from build123d import *

# Parameters (mm, degrees)
MAKERBEAMFIX_DEPTH              = 15
SKETCH3_W                       = 30
SKETCH3_H                       = 12
SKETCH3_R                       = 3.25
SKETCH3_R_2                     = 4.5
DRILLKEYANDSMALLHEXDRIVER_DEPTH = 10
SKETCH4_R                       = 1.5
FIXINGHOLE_DEPTH                = 15
SKETCH5_R                       = 4.25
DRIVERHOLE_DEPTH                = 7


with BuildPart() as part:
    # Sketch1 → MakerBeamFix (new body, symmetric)
    with BuildSketch(Plane.XY):
        Polygon((-5, 0), (5, 0), (5, 1), (1.45, 1), (1.45, 2), (-1.45, 2), (-1.45, 1), (-5, 1), align=None)
    extrude(amount=MAKERBEAMFIX_DEPTH, both=True)

    # Sketch3 → DrillKeyAndSmallHexDriver (add)
    with BuildSketch(Plane.ZY.offset(5)):
        with Locations((0, -6)):
            Rectangle(SKETCH3_W, SKETCH3_H)
        with Locations((9, -6)):
            Circle(SKETCH3_R, mode=Mode.SUBTRACT)
        with Locations((-8, -6)):
            Circle(SKETCH3_R_2, mode=Mode.SUBTRACT)
    extrude(amount=-DRILLKEYANDSMALLHEXDRIVER_DEPTH)

    # Sketch4 → FixingHole (cut, through all)
    with BuildSketch(Plane.XZ.offset(12)):
        with Locations((0, 1)):
            Circle(SKETCH4_R)
    extrude(amount=-FIXINGHOLE_DEPTH, mode=Mode.SUBTRACT)

    # Sketch5 → DriverHole (cut, through all)
    with BuildSketch(Plane(origin=(0, -6, 0), x_dir=(1, 0, 0), z_dir=(0, 1, 0))):
        with Locations((0, -1)):
            Circle(SKETCH5_R)
    extrude(amount=-DRIVERHOLE_DEPTH, mode=Mode.SUBTRACT)


solid = part.part
Geometry: final body of the model. Coordinates: model frame, mm. A direction names the side the tool comes from. Round coordinates to 2 decimals unless told otherwise and drop trailing zeros. Loops run counter-clockwise (first coordinate to the right, second up) from the corner with the lowest first, then second, coordinate; pieces in that order, holes last. Notation, with made-up numbers: (83.25, 38.25) - (139.25, 38.25) arc R21 ccw to (139.25, 69.25) - close; hole circle Ø8 at (86.5, 50.25). An arc over 180 degrees is marked (long way). Write each question's results on one line, items separated by ' | '. Start each with the question number.
1) Cut plane C-C on y = -7.75. Return loops of the section in (x, z), then the cut area to 3 significant figures.
2) Cut plane B-B on z = 1. Return loops of the section in (x, y), then the cut area to 3 significant figures.
3) Cut plane D-D on z = -8. Return loops of the section in (x, y).
4) Line query: probe 1 along Z at (x, y) = (0.5, -7.25); probe 2 along Z at (x, y) = (-4, -4.5); probe 3 along Z at (x, y) = (0.5, -8.25). Output: solid intervals per line, ascending. Write a range as [from, to].
5) First-contact query: P1, Ø3, axis at x = -2.5, z = 2.5, coming from the +Y side; P2, Ø1.1, axis at x = 4, z = 0, coming from the +Y side; P3, Ø0.8, axis at y = 1.5, z = 8, coming from the -X side; P4, Ø4, axis at x = -2, z = 0.5, coming from the -Y side. Flat tips, straight axial feed; report the tip coordinate or a pass-through.
6) Cut plane A-A on x = 0. Return loops of the section in (y, z), then the cut area to 3 significant figures.
7) Access query for faces 4 (the face through (0, -5, -15)), 5 (the face through (1.45, 1.5, 8.3)), 6 (the face through (-3, 1, 0)), 7 (the face through (-0.92, -8.96, 5.15)), 8 (the face through (0, 2, -7)). Directions: +Z, -Z, +X, -X, +Y, -Y. A direction counts if a zero-diameter tool reaches every point of the face in a straight line with its end or side. Return the directions, or none.
8) Mould query, pull axis X, two halves, no side actions, for faces 1 (the face through (1.45, 1.5, -7.1)), 2 (the face through (-1.45, 1.5, -7.1)), 3 (the face through (2, -6, 1)). Classes: released by +X, released by -X, zero draft, split by the parting line, or undercut.
Verdict:
1) outline: (-5, -15) - (5, -15) - (5, -12.15) - (-5, -12.15) - close; (-5, -3.85) - (5, -3.85) - (5, 6.26) - (-5, 6.26) - close; (-5, 11.74) - (5, 11.74) - (5, 15) - (-5, 15) - close; hole circle Ø8.5 at (0, 1) | area: 106 mm2
2) outline: (-5, -12) - (-4.25, -12) - (-4.25, -6) - (-1.5, -6) - (-1.5, 1) - (-5, 1) - close; (1.5, -6) - (4.25, -6) - (4.25, -12) - (5, -12) - (5, 1) - (1.5, 1) - close | area: 58.0 mm2
3) outline: (-5, -12) - (5, -12) - (5, -10.5) - (-5, -10.5) - close; (-5, -1.5) - (5, -1.5) - (5, 1) - (1.45, 1) - (1.45, 2) - (-1.45, 2) - (-1.45, 1) - (-5, 1) - close
4) probe 1: z = [-15, -12.32], [-3.68, -3.22], [5.22, 6], [12, 15] | probe 2: z = [-15, -12.24], [-3.76, 6.12], [11.88, 15] | probe 3: z = [-15, -11.9], [-4.1, -3.22], [5.22, 6.65], [11.35, 15]
5) P1: stops at y = 2 | P2: stops at y = 1 | P3: stops at x = -1.45 | P4: stops at y = -6
6) outline: (-12, -15) - (2, -15) - (2, -0.5) - (-6, -0.5) - (-6, -3.25) - (-12, -3.25) - close; (-12, 5.25) - (-6, 5.25) - (-6, 2.5) - (2, 2.5) - (2, 15) - (-12, 15) - close; hole circle Ø9 at (-6, -8); hole circle Ø6.5 at (-6, 9) | area: 248 mm2
7) face 4: -Z, +X, -X, +Y, -Y | face 5: +Z, -Z, +X, +Y | face 6: +Z, -Z, -X, +Y | face 7: -Y | face 8: +Z, -Z, +X, -X, +Y
8) face 1: released by +X | face 2: released by -X | face 3: undercut
